Design review of the part shown in the three views and the two pictorial views. Dimensions are in mm from the part's minimum x, y and z. Give positions to 0.01 mm unless a question says otherwise; leave off trailing zeros. Write each loop counter-clockwise with the first axis right and the second up, starting at its lowest first coordinate (ties: lowest second). Pieces come first, ordered by that corner, then holes. Notation, with made-up numbers: M 40.5,78 L 63.5,78 A7 cw 63.5,83 Z; hole C 76,-18 d6. An arc over 180 degrees is marked long. Use one line per item in the form item = value. Start each with the question number.
Q1. For probe 1 along Y at (x, z) = (100, 13.75); probe 2 along X at (y, z) = (111, 1.5); probe 3 along X at (y, z) = (156, 8.75), list the stretches that pass through material, from the lowest coordinate up. Write a range as [from, to].
Q2. Consider section A-A on y = 100. Write out the cut boundary in (x, z).
Q3. Clearance check with flat-ended pins moving along their axes: pin 1 Ø3 at (x, z) = (81.5, 16.5) entering from +Y; pin 2 Ø3 at (x, z) = (177, 18) entering from -Y; pin 3 Ø2 at (x, z) = (147, 19) entering from +Y. State where each tip first meets the part, or that it passes through.
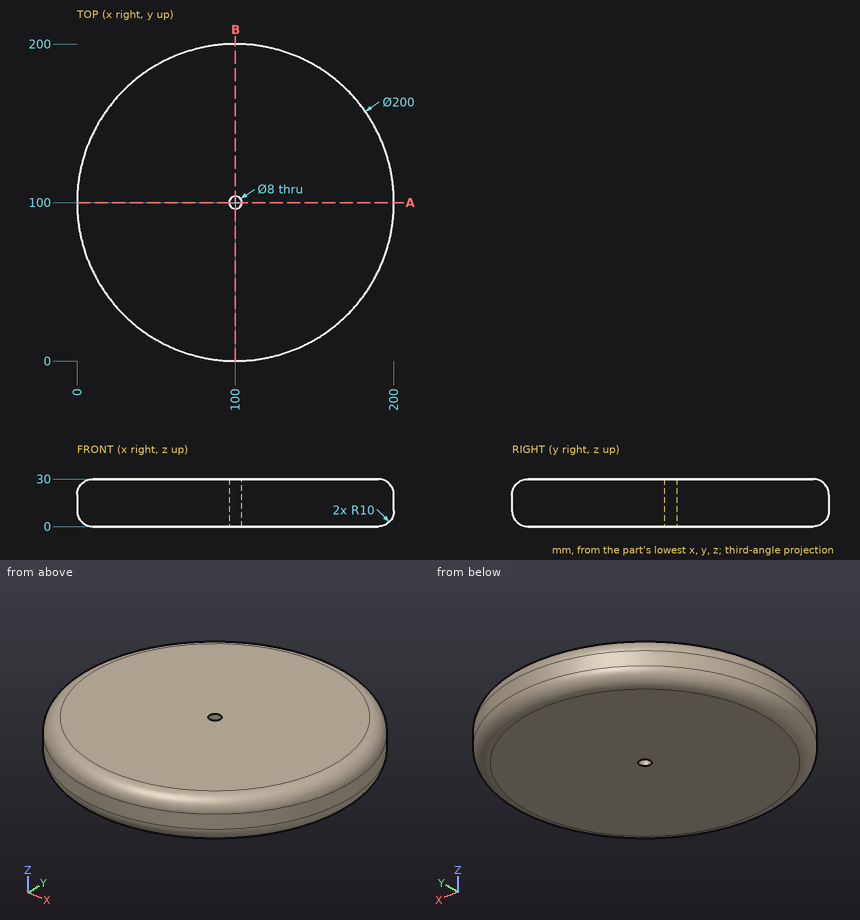
Working result:
q1.probe_1 = [0, 96], [104, 200]
q1.probe_2 = [5.37, 194.63]
q1.probe_3 = [17.25, 182.75]
q2.outline = M 0,10 A10 ccw 10,0 L 96,0 L 96,30 L 10,30 A10 ccw 0,20 Z; M 104,0 L 190,0 A10 ccw 200,10 L 200,20 A10 ccw 190,30 L 104,30 Z
q3.pin_1 = 198.54
q3.pin_2 = 34.43
q3.pin_3 = 188.79
